Here's how the part is built. I have some questions about the finished solid (model axes, mm). A direction names the side the tool comes from. Give positions to 0.01 mm unless a question says otherwise; leave off trailing zeros. Loops run counter-clockwise (first coordinate to the right, second up) from the corner with the lowest first, then second, coordinate; pieces in that order, holes last. Notation, with made-up numbers: (-15, -31) - (44, -31) arc R20 cw to (44, -20) - close; hole circle Ø10 at (43.5, 69). An arc over 180 degrees is marked (long way). Use a Markdown table: item, result.
from build123d import *

# Parameters (mm, degrees)
BASE_DEPTH            = 2.7
WHEEL_HOLE_REACH      = 54.984
SKETCH3_R             = 2.5
BATTERY_HOLDER_DEPTH  = 2.7
IR_SENSOR_DIVOT_DEPTH = 56


with BuildPart() as part:
    # Sketch1 → Base (new body)
    with BuildSketch(Plane(origin=(0, 0, 0), x_dir=(1, 0, 0), z_dir=(0, 1, 0))):
        with BuildLine():
            Line((34.641016151, 20), (34.641016151, -20))
            ThreePointArc((34.641016151, -20), (0, -40), (-34.641016151, -20))
            Line((-34.641016151, -20), (-34.641016151, 20))
            ThreePointArc((-34.641016151, 20), (0, 40), (34.641016151, 20))
        make_face()
    extrude(amount=BASE_DEPTH)

    # Sketch2 → Wheel Hole (cut, up to next)
    with BuildSketch(Plane(origin=(0, 2.7, 0), x_dir=(-1, 0, 0), z_dir=(0, 1, 0)), mode=Mode.PRIVATE) as wheel_hole_sk1:
        with BuildLine():
            Line((27.641016151, -18), (27.641016151, 18))
            ThreePointArc((27.641016151, 18), (29.641016151, 20), (31.641016151, 18))
            Line((31.641016151, 18), (31.641016151, -18))
            ThreePointArc((31.641016151, -18), (29.641016151, -20), (27.641016151, -18))
        make_face()
    wheel_hole_tool1 = extrude(wheel_hole_sk1.sketch, amount=-WHEEL_HOLE_REACH, mode=Mode.PRIVATE) & part.part
    wheel_hole = wheel_hole_tool1.solids().sort_by_distance((-29.641016, 2.7, 0))[0]
    add(wheel_hole, mode=Mode.SUBTRACT)

    # Sketch3 → Battery Holder (add)
    with BuildSketch(Plane(origin=(-20.5, 0, 0), x_dir=(0, 0, -1), z_dir=(1, 0, 0))):
        with BuildLine():
            Line((27.5, 2.7), (27.5, 10.2))
            ThreePointArc((27.5, 10.2), (20, 17.7), (12.5, 10.2))
            Line((12.5, 10.2), (12.5, 2.7))
            Line((12.5, 2.7), (27.5, 2.7))
        make_face()
        with Locations((20, 10.2)):
            Circle(SKETCH3_R, mode=Mode.SUBTRACT)
    battery_holder = extrude(amount=-BATTERY_HOLDER_DEPTH)

    # Sketch5 → IR Sensor Divot (cut, symmetric)
    with BuildSketch(Plane(origin=(0, 2.7, 0), x_dir=(-1, 0, 0), z_dir=(0, 1, 0))):
        Polygon((5, 229.919345803), (5, 39.686269666), (5, 37.986269666), (8.6, 37.986269666), (8.6, 39.064561946), (8.6, 229.297638083), (73.346792401, 604.214089975), (69.746792401, 604.835797696), align=None)
    ir_sensor_divot = extrude(amount=IR_SENSOR_DIVOT_DEPTH, both=True, mode=Mode.SUBTRACT)

    # Mirror 2: Wheel Hole, Battery Holder, IR Sensor Divot across plane
    add(wheel_hole.mirror(Plane(origin=(0, 0, 0), x_dir=(0, 0, 1), z_dir=(1, 0, 0))), mode=Mode.SUBTRACT)
    add(battery_holder.mirror(Plane(origin=(0, 0, 0), x_dir=(0, 0, 1), z_dir=(1, 0, 0))))
    add(ir_sensor_divot.mirror(Plane(origin=(0, 0, 0), x_dir=(0, 0, 1), z_dir=(1, 0, 0))), mode=Mode.SUBTRACT)


solid = part.part
(1) Suppose I cut it at B-B on y = 16.75. Write out the boundary of the cut face in (x, z), plus the area to 3 significant figures.
A:
| item | result |
|---|---|
| outline | (-23.2, -23.65) - (-20.5, -23.65) - (-20.5, -16.35) - (-23.2, -16.35) - close; (20.5, -23.65) - (23.2, -23.65) - (23.2, -16.35) - (20.5, -16.35) - close |
| area | 39.5 mm2 |
(2) If I drill on line 1 (X direction, y = 1.25, z = 17); line 2 (Y direction, x = 22.3, z = -20); line 3 (X direction, y = 14.5, z = -14.5), over which ranges is the centre line in solid material (lowest first)?
A:
| item | result |
|---|---|
| line 1 | -34.64 to -31.64, -27.64 to 27.64, 31.64 to 34.64 |
| line 2 | 0 to 7.7, 12.7 to 17.7 |
| line 3 | -23.2 to -20.5, 20.5 to 23.2 |
(3) Suppose I cut it at D-D on x = -3.5. Write out the boundary of the cut face in (y, z).
A:
| item | result |
|---|---|
| outline | (0, -39.85) - (2.7, -39.85) - (2.7, 39.85) - (0, 39.85) - close |
(4) Suppose I cut it at C-C on z = 32. Write out the boundary of the cut face in (x, y).
A:
| item | result |
|---|---|
| outline | (-24, 0) - (24, 0) - (24, 2.7) - (-24, 2.7) - close |
(5) Will these pins go through, and if not, where does the flat tip stop? pin 1 (4.5 mm diameter, centred on y = 10.2, z = -20, fed in from -X); pin 2 (1 mm diameter, centred on x = -21, z = 26.5, fed in from +Y); pin 3 (1.3 mm diameter, centred on x = -22, y = 7.5, fed in from +Z); pin 4 (7.5 mm diameter, centred on y = 9, z = -19.5, fed in from -X).
A:
| item | result |
|---|---|
| pin 1 | through |
| pin 2 | y = 2.7 |
| pin 3 | z = -12.5 |
| pin 4 | x = -23.2 |
(6) On a 3-axis mill with a long thin cutter (end or side, diameter ignored), from which of +Z, -Z, +X, -X, +Y, -Y can I reach the whole of each face in a straight line? I mean faces 1 (the face through (21.8, 10.3, -17.5)), 2 (the face through (-23.2, 7, -20)), 3 (the face through (7, 1, 37.986)), 4 (the face through (22, 7, -12.5)), 5 (the face through (27.641, 1, 0)). Say none if no direction works.
A:
| item | result |
|---|---|
| face 1 | +X, -X |
| face 2 | +Z, -Z, -X, +Y |
| face 3 | +Z, +Y, -Y |
| face 4 | +Z, +X, -X, +Y |
| face 5 | +Y, -Y |
(7) We'd pull the mould along Z, two halves only. Please class faces 6 (the face through (-0.586, 1.331, -39.996)), 7 (the face through (-22, 7, -12.5)), 8 (the face through (-29.7, 1.4, -20)): pulls with the +Z half, pulls with the -Z half, needs draft (parallel to the pull), parting line crosses it, or undercut.
A:
| item | result |
|---|---|
| face 6 | pulls with the -Z half |
| face 7 | pulls with the +Z half |
| face 8 | undercut |
(8) Suppose I cut it at A-A on x = -22. Write out the boundary of the cut face in (y, z), plus the area to 3 significant figures.
A:
| item | result |
|---|---|
| outline | (0, -33.41) - (2.7, -33.41) - (2.7, -27.5) - (10.2, -27.5) arc R7.5 ccw to (10.2, -12.5) - (2.7, -12.5) - (2.7, 33.41) - (0, 33.41) - close; hole circle Ø5 at (10.2, -20) |
| area | 362 mm2 |
